Read the model definition and answer for the solid it produces. Units are mm, in the model's axes. Give positions to 0.01 mm unless a question says otherwise; leave off trailing zeros. Order: outer loops, then holes, each group sorted by start corner. A loop starts at its lowest first (then second) coordinate and runs counter-clockwise, first axis right, second up.
```python
from build123d import *

# Parameters (mm, degrees)
SKETCH_R    = 8.5
SKETCH_R_2  = 3
PAD_DEPTH   = 3
SKETCH001_R = 3.05
HOLE_DEPTH  = 3.001
FILLET_R    = 10


with BuildPart() as part:
    # Sketch → Pad (new body)
    with BuildSketch(Plane.XY):
        Polygon((0, 350), (-332.869781, 108.155948), (-205.724838, -283.155948), (205.724838, -283.155948), (332.869781, 108.155948), align=None)
        with Locations((0, -222.705098)):
            Circle(SKETCH_R, mode=Mode.SUBTRACT)
        with Locations((-192.868273, 111.352549)):
            Circle(SKETCH_R, mode=Mode.SUBTRACT)
        with Locations((192.868273, 111.352549)):
            Circle(SKETCH_R, mode=Mode.SUBTRACT)
        with Locations((-176.335576, -242.705098)):
            Circle(SKETCH_R_2, mode=Mode.SUBTRACT)
        with Locations((176.335576, -242.705098)):
            Circle(SKETCH_R_2, mode=Mode.SUBTRACT)
        with Locations((285.316955, 92.705098)):
            Circle(SKETCH_R_2, mode=Mode.SUBTRACT)
        with Locations((-285.316955, 92.705098)):
            Circle(SKETCH_R_2, mode=Mode.SUBTRACT)
        with Locations((0, 300)):
            Circle(SKETCH_R_2, mode=Mode.SUBTRACT)
    extrude(amount=PAD_DEPTH)

    # Sketch001 (on Face15 of Pad) → Hole (cut, through all)
    with BuildSketch(Plane.XY.offset(3)):
        with Locations((-38.206041, 52.586105)):
            Circle(SKETCH001_R)
        with Locations((38.206041, 52.586105)):
            Circle(SKETCH001_R)
        with Locations((0, -65)):
            Circle(SKETCH001_R)
        Circle(SKETCH001_R)
    extrude(amount=-HOLE_DEPTH, mode=Mode.SUBTRACT)

    # Fillet
    fillet_edges = [part.edges().sort_by_distance(p)[0] for p in [
        (-332.869781, 108.155948, 1.5),
        (0, 350, 1.5),
        (332.869781, 108.155948, 1.5),
        (205.724838, -283.155948, 1.5),
        (-205.724838, -283.155948, 1.5),
    ]]
    fillet(fillet_edges, radius=FILLET_R)


solid = part.part
```
1) The part is cut by section B-B on y = -190. Determine the outline of the cut face in (x, z), and give its area (3 significant figures).
Final values:
outline: (-235.99, 0) - (235.99, 0) - (235.99, 3) - (-235.99, 3) - close
area: 1,420 mm2
2) Consider L1, parallel to Y at x = 0, z = 1.7; L2, parallel to X at y = 300, z = 1.65; L3, parallel to X at y = 109.5, z = 2.5. Determine where each line is inside the solid, lowest interval first.
Final values:
L1: y = -283.16 to -231.21, -214.21 to -68.05, -61.95 to -3.05, 3.05 to 297, 303 to 347.64
L2: x = -68.82 to -3, 3 to 68.82
L3: x = -329.68 to -201.16, -184.57 to 184.57, 201.16 to 329.68
3) The part is cut by section C-C on x = 63. Determine the outline of the cut face in (y, z), and give its area (3 significant figures).
Final values:
outline: (-283.16, 0) - (304.23, 0) - (304.23, 3) - (-283.16, 3) - close
area: 1,760 mm2
4) The part is cut by section A-A on z = 2. Count the separate pieces of the cut face and the enclosed holes in it, and give its area (3 significant figures).
Final values:
separate pieces: 1
enclosed holes: 12
area: 290,000 mm2
5) Given pin 1 (1.5 mm diameter, centred on x = 51.5, z = 1, fed in from +Y), flat-ended and moving along its own axis, determine where the tip first touches the part or whether it passes through.
Final values:
pin 1: stops at y = 313.13
6) For a pull along Y with two mould halves and no side action, classify faces 1 (the face through (-164.2, 230.7, 1.5)), 2 (the face through (191.026, 103.055, 1.479)), 3 (the face through (268.44, -90.14, 1.48)), 4 (the face through (-199.614, 106.18, 1.479)) as released by +Y, released by -Y, zero draft, split by the parting line, or undercut.
Final values:
face 1: released by +Y
face 2: undercut
face 3: released by -Y
face 4: undercut
